Model file for the job. Use its own axes, mm. A direction names the side the tool comes from. Round coordinates to 2 decimals unless told otherwise and drop trailing zeros. Write each loop counter-clockwise with the first axis right and the second up, starting at its lowest first coordinate (ties: lowest second). Pieces come first, ordered by that corner, then holes. Notation, with made-up numbers: (75.25, -6.75) - (103.25, -6.75) arc R11 ccw to (103.25, 7.25) - close; hole circle Ø9 at (-18.5, -22.5). An arc over 180 degrees is marked (long way). Answer as a JSON object with one key per item and string values. Group by question number.
from build123d import *

# Parameters (mm, degrees)
BOSS_EXTRUDE1_DEPTH = 2


with BuildPart() as part:
    # Sketch1 → Boss-Extrude1 (new body)
    with BuildSketch(Plane(origin=(0, 0, 0), x_dir=(1, 0, 0), z_dir=(0, 1, 0))):
        Polygon((0, 0), (15.84078026, 0), (13.860874637, 11.718342674), (2.63902101, 15.619407394), align=None)
        Polygon((5.005894234, 11.620506435), (3.549392266, 3), (12.291387994, 3), (11.198615402, 9.467724294), align=None, mode=Mode.SUBTRACT)
    extrude(amount=BOSS_EXTRUDE1_DEPTH)


solid = part.part
(1) 3-axis set-ups, long thin cutter, end or side, ignore diameter. For faces 1 (the flat face through (8.146, 0.986, -10.529)), 2 (the flat face through (8.33, 0.99, -13.64)): which of +Z, -Z, +X, -X, +Y, -Y reach the whole face in a straight line?
(2) Slice it at D-D (z = -13.75). Write the cut outline in (x, y), then the cut area to 3 significant figures.
(3) Flat gauge pins, fed straight in: pin 1 (1 mm diameter, centred on y = 0.5, z = -1.5, fed in from -X); pin 2 (1 mm diameter, centred on y = 1.5, z = -6.5, fed in from +X); pin 3 (1 mm diameter, centred on x = 7, y = 1, fed in from -Z). Where does each tip first touch, or does it go through?
(4) Slice it at B-B (z = -4.5). Write the cut outline in (x, y).
(5) Slice it at A-A (y = 0.5). Write the cut outline in (x, z), then the cut area to 3 significant figures.
(6) Slice it at C-C (x = 10.5). Write the cut outline in (y, z).
(7) Pull direction Z, two halves, no side cores. Call faces 3 (the flat face through (14.865, 0.986, -5.777)), 4 (the flat face through (4, 0, -8)), 5 (the flat face through (4.288, 0.986, -7.371)): pulls with the +Z half, pulls with the -Z half, needs draft (parallel to the pull), parting line crosses it, or undercut.
(8) Drill centre lines: line 1 (Z direction, x = 7, y = 0.65); line 2 (Z direction, x = 9, y = 1.65); line 3 (X direction, y = 0.85, z = -7.5). Where is each one in solid material? Low to high. Write a range as from..to.
Answer:
{
 "1": {"face 1": "+Y, -Y", "face 2": "-Z, +X, +Y, -Y"},
 "2": {"outline": "(2.32, 0) - (8.02, 0) - (8.02, 2) - (2.32, 2) - close", "area": "11.4 mm²"},
 "3": {"pin 1": "x = 0.17", "pin 2": "x = 14.83", "pin 3": "z = -14.28"},
 "4": {"outline": "(0.76, 0) - (3.8, 0) - (3.8, 2) - (0.76, 2) - close; (12.04, 0) - (15.08, 0) - (15.08, 2) - (12.04, 2) - close"},
 "5": {"outline": "(0, 0) - (2.64, -15.62) - (13.86, -11.72) - (15.84, 0) - close; hole (3.55, -3) - (5.01, -11.62) - (11.2, -9.47) - (12.29, -3) - close", "area": "129 mm²"},
 "6": {"outline": "(0, -12.89) - (2, -12.89) - (2, -9.71) - (0, -9.71) - close; (0, -3) - (2, -3) - (2, 0) - (0, 0) - close"},
 "7": {"face 3": "pulls with the -Z half", "face 4": "needs draft", "face 5": "undercut"},
 "8": {"line 1": "-14.1..-10.93, -3..0", "line 2": "-13.41..-10.23, -3..0", "line 3": "1.27..4.31, 11.53..14.57"}
}
